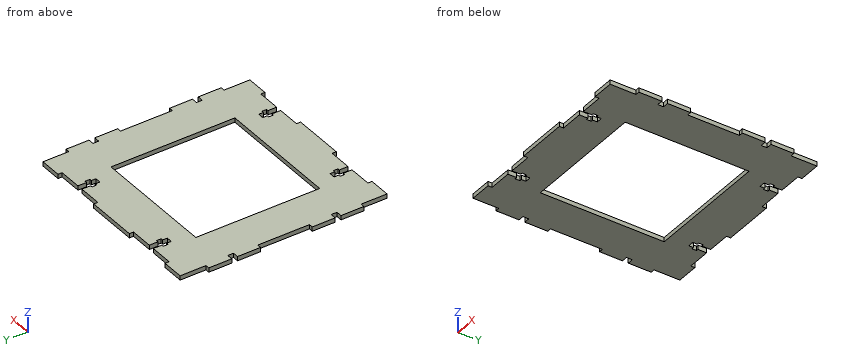
from build123d import *

# Parameters (mm, degrees)
SKETCH1_W           = 89.973098965
SKETCH1_H           = 90.646237782
BOSS_EXTRUDE1_DEPTH = 3.175


with BuildPart() as part:
    # Sketch1 → Boss-Extrude1 (new body)
    with BuildSketch(Plane.XY):
        Polygon((157.378148634, 154.39750188), (157.378148634, 135.470394989), (154.39750188, 135.470394989), (154.39750188, 118.65457955), (158.620084782, 118.65457955), (158.620084782, 116.543288099), (158.620084782, 114.431996648), (154.39750188, 114.431996648), (154.39750188, 97.616181208), (157.378148634, 97.616181208), (157.378148634, 59.761967427), (154.39750188, 59.761967427), (154.39750188, 42.946151987), (158.620084782, 42.946151987), (158.620084782, 40.834860536), (158.620084782, 38.723569085), (154.39750188, 38.723569085), (154.39750188, 21.907753645), (157.378148634, 21.907753645), (157.378148634, 2.980646754), (173.324608771, 2.980646754), (173.324608771, 5.961293509), (190.14042421, 5.961293509), (190.14042421, 12.270329139), (188.650100833, 12.270329139), (188.650100833, 15.698072907), (190.14042421, 15.698072907), (190.14042421, 19.125816674), (194.363007113, 19.125816674), (194.363007113, 15.698072907), (195.85333049, 15.698072907), (195.85333049, 12.270329139), (194.363007113, 12.270329139), (194.363007113, 5.961293509), (211.178822552, 5.961293509), (211.178822552, 2.980646754), (249.033036334, 2.980646754), (249.033036334, 5.961293509), (265.848851773, 5.961293509), (265.848851773, 12.270329139), (264.358528396, 12.270329139), (264.358528396, 15.698072907), (265.848851773, 15.698072907), (265.848851773, 19.125816674), (270.071434675, 19.125816674), (270.071434675, 15.698072907), (271.561758053, 15.698072907), (271.561758053, 12.270329139), (270.071434675, 12.270329139), (270.071434675, 5.961293509), (286.887250115, 5.961293509), (286.887250115, 2.980646754), (302.833710251, 2.980646754), (302.833710251, 21.907753645), (305.814357006, 21.907753645), (305.814357006, 38.723569085), (301.591774104, 38.723569085), (301.591774104, 40.834860536), (301.591774104, 42.946151987), (305.814357006, 42.946151987), (305.814357006, 59.761967427), (302.833710251, 59.761967427), (302.833710251, 97.616181208), (305.814357006, 97.616181208), (305.814357006, 114.431996648), (301.591774104, 114.431996648), (301.591774104, 116.543288099), (301.591774104, 118.65457955), (305.814357006, 118.65457955), (305.814357006, 135.470394989), (302.833710251, 135.470394989), (302.833710251, 154.39750188), (286.887250115, 154.39750188), (286.887250115, 151.416855126), (270.071434675, 151.416855126), (270.071434675, 145.107819495), (271.561758053, 145.107819495), (271.561758053, 141.680075728), (270.071434675, 141.680075728), (270.071434675, 138.25233196), (265.848851773, 138.25233196), (265.848851773, 141.680075728), (264.358528396, 141.680075728), (264.358528396, 145.107819495), (265.848851773, 145.107819495), (265.848851773, 151.416855126), (249.033036334, 151.416855126), (249.033036334, 154.39750188), (211.178822552, 154.39750188), (211.178822552, 151.416855126), (194.363007113, 151.416855126), (194.363007113, 145.107819495), (195.85333049, 145.107819495), (195.85333049, 141.680075728), (194.363007113, 141.680075728), (194.363007113, 138.25233196), (190.14042421, 138.25233196), (190.14042421, 141.680075728), (188.650100833, 141.680075728), (188.650100833, 145.107819495), (190.14042421, 145.107819495), (190.14042421, 151.416855126), (173.324608771, 151.416855126), (173.324608771, 154.39750188), align=None)
        with Locations((230.132306119, 78.423957663)):
            Rectangle(SKETCH1_W, SKETCH1_H, mode=Mode.SUBTRACT)
    extrude(amount=BOSS_EXTRUDE1_DEPTH)


solid = part.part
Source: CAD feature listing. Evaluate the final solid. Frame: model axes, mm. Give positions to 0.01 mm unless a question says otherwise; leave off trailing zeros. Write each loop counter-clockwise with the first axis right and the second up, starting at its lowest first coordinate (ties: lowest second). Pieces come first, ordered by that corner, then holes. Notation, with made-up numbers: (-29, -0.5) -> (26, -0.5) arc R17 cw to (26, 30.5) -> close; hole circle Ø4 at (70.25, -22). An arc over 180 degrees is marked (long way). Write item = value, one per line.
Q1. Cut plane B-B on x = 214. Return loops of the section in (y, z) (1 decimal).
Here are the results:
outline = (3, 0) -> (33.1, 0) -> (33.1, 3.2) -> (3, 3.2) -> close; (123.7, 0) -> (154.4, 0) -> (154.4, 3.2) -> (123.7, 3.2) -> close
Q2. First-contact query: pin 1 (1.6 mm diameter, centred on y = 40.5, z = 1, fed in from +X); pin 2 (1.6 mm diameter, centred on x = 156, z = 1, fed in from +Y); pin 3 (0.9 mm diameter, centred on x = 156.5, z = 1, fed in from -Y). Flat tips, straight axial feed; report the tip coordinate or a pass-through.
Here are the results:
pin_1 = 301.59
pin_2 = 135.47
pin_3 = 21.91
Q3. Cut plane C-C on x = 175.5. Return loops of the section in (y, z) (3 decimals).
Here are the results:
outline = (5.961, 0) -> (151.417, 0) -> (151.417, 3.175) -> (5.961, 3.175) -> close
Q4. Cut plane A-A on y = 108.5. Return loops of the section in (x, z) (1 decimal), then the cut area to 3 significant figures.
Here are the results:
outline = (154.4, 0) -> (185.1, 0) -> (185.1, 3.2) -> (154.4, 3.2) -> close; (275.1, 0) -> (305.8, 0) -> (305.8, 3.2) -> (275.1, 3.2) -> close
area = 195 mm²
Q5. Line query: line 1 (X direction, y = 147, z = 2.8); line 2 (Y direction, x = 269.5, z = 2.7); line 3 (Y direction, x = 245, z = 2.75). Output: solid intervals per line, ascending. Write a range as from..to.
Here are the results:
line_1 = 157.38..190.14, 194.36..265.85, 270.07..302.83
line_2 = 19.13..33.1, 123.75..138.25
line_3 = 2.98..33.1, 123.75..154.4
